Input: part model. Units: mm. Frame: model coordinates. A direction names the side the tool comes from. Give positions to 0.01 mm unless a question says otherwise; leave off trailing zeros. Loops run counter-clockwise (first coordinate to the right, second up) from the corner with the lowest first, then second, coordinate; pieces in that order, holes last. Notation, with made-up numbers: (-19.5, -39.5) -> (16.5, -39.5) arc R37 ccw to (16.5, -1.5) -> close; hole circle Ø5 at (-34, -39.5). An arc over 180 degrees is marked (long way). Answer in a Markdown table with one row per item. Add a question column.
```python
from build123d import *

# Parameters (mm, degrees)
F0_R     = 76.2734110289
F1_DEPTH = 127
F2_R     = 63.3841593345
F3_DEPTH = 63.5
F5_DEPTH = 127
F6_R     = 19.1908924799
F7_DEPTH = 102.616


with BuildPart() as f1:
    # F0 (on Top) → F1 (new body)
    with BuildSketch(Plane.XY):
        Circle(F0_R)
    extrude(amount=F1_DEPTH)

    # F2 (on face) → F3 (cut)
    with BuildSketch(Plane.XY.offset(127)):
        Circle(F2_R)
    extrude(amount=-F3_DEPTH, mode=Mode.SUBTRACT)

    # F4 (on Front) → F5 (cut)
    with BuildSketch(Plane.XZ):
        with BuildLine():
            ThreePointArc((-23.6000716686, 88.9091379941), (-27.3653091558, 79.819050587), (-36.4553965628, 76.0538130999))
            Line((-36.4553965628, 76.0538130999), (40.0476576165, 76.0538130999))
            ThreePointArc((40.0476576165, 76.0538130999), (28.1651377987, 88.9091379941), (40.0476576165, 101.7644628882))
            Line((40.0476576165, 101.7644628882), (-36.4553965628, 101.7644628882))
            ThreePointArc((-36.4553965628, 101.7644628882), (-27.3653091558, 97.9992254011), (-23.6000716686, 88.9091379941))
        make_face()
        with BuildLine():
            ThreePointArc((-36.4553965628, 101.7644628882), (-49.310721457, 88.9091379941), (-36.4553965628, 76.0538130999))
            Line((-36.4553965628, 76.0538130999), (-36.4553965628, 101.7644628882))
        make_face()
        with BuildLine():
            Line((-36.4553965628, 101.7644628882), (-36.4553965628, 76.0538130999))
            ThreePointArc((-36.4553965628, 76.0538130999), (-27.3653091558, 79.819050587), (-23.6000716686, 88.9091379941))
            ThreePointArc((-23.6000716686, 88.9091379941), (-27.3653091558, 97.9992254011), (-36.4553965628, 101.7644628882))
        make_face()
        with BuildLine():
            ThreePointArc((40.0476576165, 101.7644628882), (28.1651377987, 88.9091379941), (40.0476576165, 76.0538130999))
            Line((40.0476576165, 76.0538130999), (41.0602837801, 76.0538130999))
            Line((41.0602837801, 76.0538130999), (41.0602837801, 101.7644628882))
            Line((41.0602837801, 101.7644628882), (40.0476576165, 101.7644628882))
        make_face()
        with BuildLine():
            Line((41.0602837801, 76.0538130999), (40.0476576165, 76.0538130999))
            ThreePointArc((40.0476576165, 76.0538130999), (49.8131926588, 79.4396408562), (53.9554297615, 88.9091379941))
            ThreePointArc((53.9554297615, 88.9091379941), (49.8131926588, 98.3786351319), (40.0476576165, 101.7644628882))
            Line((40.0476576165, 101.7644628882), (41.0602837801, 101.7644628882))
            Line((41.0602837801, 101.7644628882), (41.0602837801, 76.0538130999))
        make_face()
    extrude(amount=-F5_DEPTH, mode=Mode.SUBTRACT)

    # F6 (on Front) → F7 (join)
    with BuildSketch(Plane.XZ):
        with Locations((0, 90.2522355318)):
            Circle(F6_R)
    extrude(amount=F7_DEPTH)


solid = f1.part
```
1) Material intervals for line 1 along X through (y, z) = (-2, 107); line 2 along Y through (x, z) = (0, 112); line 3 along Z through (x, y) = (52.5, -22), sorted ascending.
2) Pull-direction query (Y, two-part tool) for faces 1 (the face through (0, -102.616, 91)), 2 (the face through (-1, 1, 63.5)), 3 (the face through (11, 63, 127)); classes: +Y half, -Y half, draft (parallel to the pull), parting line (faces both ways), or undercut.
3) Section B-B on y = -43. Output: boundary loops of the cut face in (x, z).
4) Section C-C on z = 84. Output: boundary loops of the cut face in (x, y).
5) Reachability of faces 4 (the face through (-4.16, -31.272, 71.518)), 5 (the face through (-19.172, -88.016, 91.096)), 6 (the face through (0, 0, 91)) from +Z, -Z, +X, -X, +Y, -Y: full face, straight path, thin tool, end or side. Return the list, or none.
6) Pin query (flat end, axial travel): pin 1 (5 mm diameter, centred on y = 44, z = 81, fed in from +X); pin 2 (19 mm diameter, centred on x = -2.5, z = 88, fed in from +Y); pin 3 (1.5 mm diameter, centred on y = 12.5, z = 96.5, fed in from -X). Return the tip coordinate at first contact, or that it passes through.
7) Section A-A on x = 0. Output: boundary loops of the cut face in (y, z), and give its area (3 significant figures).
8) Section D-D on x = -33. Output: boundary loops of the cut face in (y, z).
Working result:
| question | item | result |
|---|---|---|
| 1 | line 1 | x = -76.25 to -63.35, -9.37 to 9.37, 63.35 to 76.25 |
| 1 | line 2 | y = -76.27 to -63.38, 63.38 to 76.27 |
| 1 | line 3 | z = 0 to 63.5 |
| 2 | face 1 | -Y half |
| 2 | face 2 | undercut |
| 2 | face 3 | draft |
| 3 | outline | (-63, 0) -> (63, 0) -> (63, 127) -> (46.57, 127) -> (46.57, 63.5) -> (-46.57, 63.5) -> (-46.57, 127) -> (-63, 127) -> close; circle Ø38.38 at (0, 90.25) |
| 4 | outline | (-48.34, 41) -> (-48.34, 59) arc R76.27 ccw to (-18.14, -74.08) -> (-18.14, -102.62) -> (18.14, -102.62) -> (18.14, -74.08) arc R76.27 ccw to (52.98, 54.87) -> (52.98, 34.79) arc R63.38 cw to (18.14, -60.73) -> (18.14, 0) -> (-18.14, 0) -> (-18.14, -60.73) arc R63.38 cw to start |
| 5 | face 4 | none |
| 5 | face 5 | -Y |
| 5 | face 6 | +Z |
| 6 | pin 1 | stops at x = 64 |
| 6 | pin 2 | stops at y = 0 |
| 6 | pin 3 | stops at x = -75.36 |
| 7 | outline | (-102.62, 71.06) -> (-76.27, 71.06) -> (-76.27, 0) -> (76.27, 0) -> (76.27, 76.05) -> (63.38, 76.05) -> (63.38, 63.5) -> (-63.38, 63.5) -> (-63.38, 71.06) -> (0, 71.06) -> (0, 109.44) -> (-63.38, 109.44) -> (-63.38, 127) -> (-76.27, 127) -> (-76.27, 109.44) -> (-102.62, 109.44) -> close; (63.38, 101.76) -> (76.27, 101.76) -> (76.27, 127) -> (63.38, 127) -> close |
| 7 | area | 14,400 mm2 |
| 8 | outline | (-68.77, 0) -> (68.77, 0) -> (68.77, 76.05) -> (54.12, 76.05) -> (54.12, 63.5) -> (-54.12, 63.5) -> (-54.12, 127) -> (-68.77, 127) -> close; (54.12, 101.76) -> (68.77, 101.76) -> (68.77, 127) -> (54.12, 127) -> close |
